Work out the finished part from the listing and answer in its coordinate system (mm). A direction names the side the tool comes from. Coordinates: 2 decimals unless noted, no trailing zeros. Use a Markdown table: item, result. Add a question column.
(1) The part is cut by section A-A, the plane z = -100.5. State how many separate pieces and enclosed holes the cut face has, then the cut area to 3 significant figures.
(2) Find the intervals of material crossed by line 1 (Y direction, x = 8.1, z = -120.65) (3 decimals); line 2 (X direction, y = -7.9, z = 120.65) (3 decimals); line 3 (X direction, y = 6.25, z = 116.5) (3 decimals), in increasing order. Write a range as from..to.
(3) Given pin 1 Ø3 at (y, z) = (5.5, 101.5) entering from -X; pin 2 Ø10 at (x, y) = (0, 5.5) entering from -Z, each flat-ended and moving along its own axis, determine where each tip first touches the part or whether it passes through.
(4) A tool of negligible diameter and unlimited length cuts with its end or side. For faces 1 (the face through (9.525, -2, 2)), 2 (the face through (1, -6.35, 2)), from which of +Z, -Z, +X, -X, +Y, -Y can it reach the whole face along a straight path? Write none if from no direction.
from build123d import *

# Parameters (mm, degrees)
BOSS_EXTRUDE1_DEPTH = 133.35
SKETCH3_R           = 1.651
CUT_EXTRUDE1_DEPTH  = 135.628985549
SKETCH4_R           = 1.651
CUT_EXTRUDE2_DEPTH  = 135.628985549
CUT_EXTRUDE3_DEPTH  = 135.628985549
LPATTERN1_COUNT     = 5
LPATTERN1_PITCH     = 48.26
CUT_EXTRUDE4_DEPTH  = 135.628985549
LPATTERN2_COUNT     = 5
LPATTERN2_PITCH     = 48.26


with BuildPart() as part:
    # Sketch2 → Boss-Extrude1 (new, symmetric)
    with BuildSketch(Plane.XY):
        with BuildLine():
            Line((-9.525, -9.525), (9.525, -9.525))
            Line((9.525, -9.525), (9.525, 9.525))
            Line((9.525, 9.525), (7.9375, 9.525))
            ThreePointArc((7.9375, 9.525), (6.814967985, 9.060032015), (6.35, 7.9375))
            Line((6.35, 7.9375), (6.35, -3.175))
            ThreePointArc((6.35, -3.175), (5.42006403, -5.42006403), (3.175, -6.35))
            Line((3.175, -6.35), (-7.9375, -6.35))
            ThreePointArc((-7.9375, -6.35), (-9.060032015, -6.814967985), (-9.525, -7.9375))
            Line((-9.525, -7.9375), (-9.525, -9.525))
        make_face()
    extrude(amount=BOSS_EXTRUDE1_DEPTH, both=True)

    # Sketch3 → Cut-Extrude1 (cut, through all)
    with BuildSketch(Plane(origin=(0, -6.35, 0), x_dir=(1, 0, 0), z_dir=(0, 1, 0))):
        with Locations(Location((-2.38125, 127, 0), (0, 0, 180))):
            Circle(SKETCH3_R)
        with Locations(Location((-2.38125, 120.65, 0), (0, 0, 180))):
            Circle(SKETCH3_R)
        with Locations((-2.38125, -120.65)):
            Circle(SKETCH3_R)
        with Locations((-2.38125, -127)):
            Circle(SKETCH3_R)
    extrude(amount=-CUT_EXTRUDE1_DEPTH, mode=Mode.SUBTRACT)

    # Sketch4 → Cut-Extrude2 (cut, through all)
    with BuildSketch(Plane.ZY.offset(-6.35)):
        with Locations(Location((-127, 2.381250687, 0), (0, 0, 270))):
            Circle(SKETCH4_R)
        with Locations(Location((-120.650000001, 2.381165043, 0), (0, 0, 270))):
            Circle(SKETCH4_R)
        with Locations(Location((120.650000001, 2.381165043, 0), (0, 0, 90))):
            Circle(SKETCH4_R)
        with Locations(Location((127, 2.381250687, 0), (0, 0, 90))):
            Circle(SKETCH4_R)
    extrude(amount=-CUT_EXTRUDE2_DEPTH, mode=Mode.SUBTRACT)

    # Sketch5 → Cut-Extrude3 (cut, through all)
    with BuildSketch(Plane.ZY.offset(-6.35)):
        with BuildLine():
            Line((-107.950000001, 5.556165043), (-82.550000001, 5.556165043))
            ThreePointArc((-82.550000001, 5.556165043), (-79.375000001, 2.381165043), (-82.550000001, -0.793834957))
            Line((-82.550000001, -0.793834957), (-107.950000001, -0.793834957))
            ThreePointArc((-107.950000001, -0.793834957), (-111.125000001, 2.381165043), (-107.950000001, 5.556165043))
        make_face()
    cut_extrude3 = extrude(amount=-CUT_EXTRUDE3_DEPTH, mode=Mode.SUBTRACT)

    # LPattern1: Cut-Extrude3 ×5
    with Locations(*[(0, 0, i * LPATTERN1_PITCH) for i in range(1, LPATTERN1_COUNT)]):
        add(cut_extrude3, mode=Mode.SUBTRACT)

    # Sketch6 → Cut-Extrude4 (cut, through all)
    with BuildSketch(Plane(origin=(0, -6.35, 0), x_dir=(1, 0, 0), z_dir=(0, 1, 0))):
        with BuildLine():
            Line((-5.55625, 107.95), (-5.55625, 82.55))
            ThreePointArc((-5.55625, 82.55), (-2.38125, 79.375), (0.79375, 82.55))
            Line((0.79375, 82.55), (0.79375, 107.95))
            ThreePointArc((0.79375, 107.95), (-2.38125, 111.125), (-5.55625, 107.95))
        make_face()
    cut_extrude4 = extrude(amount=-CUT_EXTRUDE4_DEPTH, mode=Mode.SUBTRACT)

    # LPattern2: Cut-Extrude4 ×5
    with Locations(*[(0, 0, i * LPATTERN2_PITCH) for i in range(1, LPATTERN2_COUNT)]):
        add(cut_extrude4, mode=Mode.SUBTRACT)


solid = part.part
Model answer:
| question | item | result |
|---|---|---|
| 1 | separate pieces | 3 |
| 1 | enclosed holes | 0 |
| 1 | area | 71.6 mm^2 |
| 2 | line 1 | -9.525..0.73, 4.032..9.525 |
| 2 | line 2 | -9.525..-4.032, -0.73..9.525 |
| 2 | line 3 | 6.35..9.525 |
| 3 | pin 1 | x = 6.35 |
| 3 | pin 2 | through |
| 4 | face 1 | +Z, -Z, +X, +Y, -Y |
| 4 | face 2 | +Z, -Z, -X, +Y |
